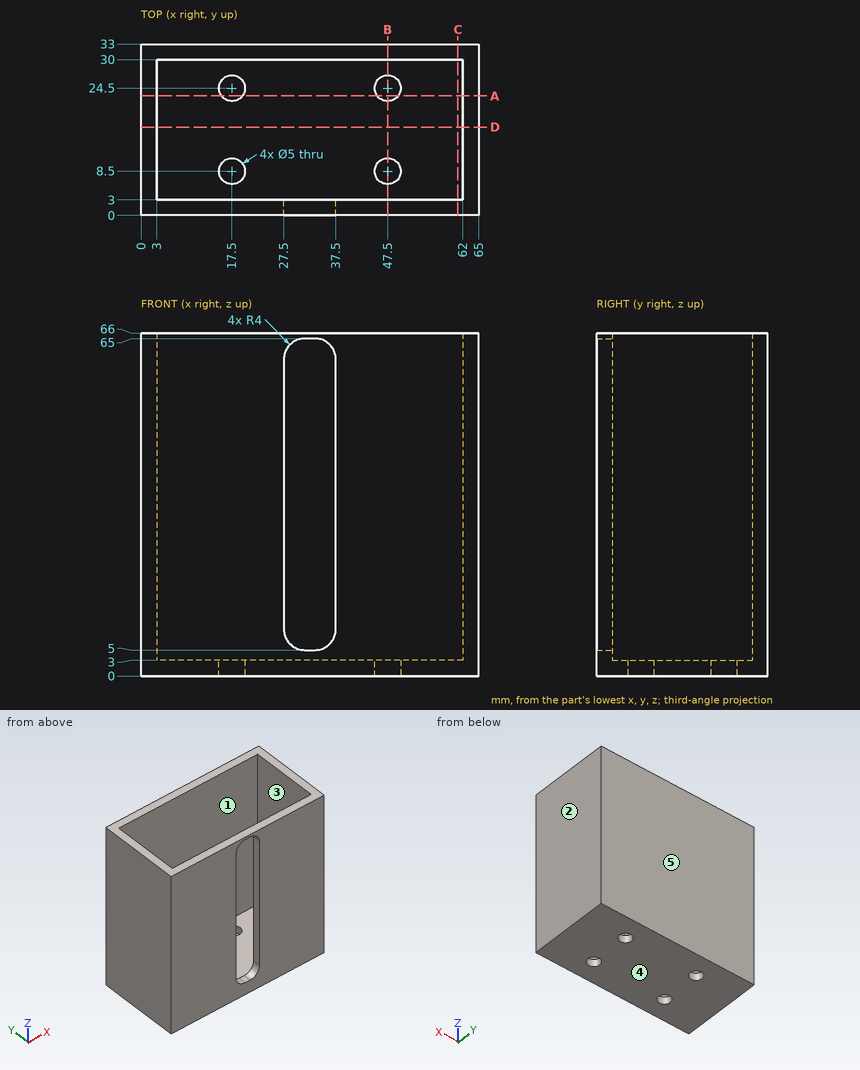
Print and shaded views of the part. All mm, measured from the part's lowest x, y and z. A direction names the side the tool comes from. Round coordinates to 2 decimals unless told otherwise and drop trailing zeros. Write each loop counter-clockwise with the first axis right and the second up, starting at its lowest first coordinate (ties: lowest second). Pieces come first, ordered by that corner, then holes. Notation, with made-up numbers: (83.5, 13) -> (131.5, 13) arc R33 ccw to (131.5, 51) -> close; hole circle Ø7 at (-10.75, 88). An arc over 180 degrees is marked (long way). Return JSON: item names as keys, results as strings. Group by question number.
Q1. Pin check, flat tips, straight feed: pin 1 (8 mm diameter, centred on x = 47.5, y = 24.5, fed in from +Z); pin 2 (4.5 mm diameter, centred on x = 47.5, y = 8.5, fed in from -Z). Stop position of each tip, or through.
Q2. Saw through at D-D on y = 17. Write the cut outline in (x, z).
Q3. Saw through at A-A on y = 23. Write the cut outline in (x, z), plus the area to 3 significant figures.
Q4. Saw through at B-B on x = 47.5. Write the cut outline in (y, z).
Q5. Saw through at C-C on x = 61. Write the cut outline in (y, z).
Q6. Which spindle directions (+Z, -Z, +X, -X, +Y, -Y) get a long thin tool onto all of the face, cutting with end or side? Do the marked faces 1 and 2. Say none if no direction does.
Q7. Mould opens along Y. For the marked faces 3, 4 and 5 say: pulls with the +Y half, pulls with the -Y half, needs draft (parallel to the pull), parting line crosses it, or undercut.
Q8. Probe L1, parallel to Y at x = 17.5, z = 2.1; L2, parallel to X at y = 27.5, z = 37; L3, parallel to Y at x = 47, z = 1. List the from-to ranges inside material, lowest first. Write a range as [from, to].
Answer:
{
 "1": {"pin 1": "z = 3", "pin 2": "through"},
 "2": {"outline": "(0, 0) -> (65, 0) -> (65, 66) -> (62, 66) -> (62, 3) -> (3, 3) -> (3, 66) -> (0, 66) -> close"},
 "3": {"outline": "(0, 0) -> (15.5, 0) -> (15.5, 3) -> (3, 3) -> (3, 66) -> (0, 66) -> close; (19.5, 0) -> (45.5, 0) -> (45.5, 3) -> (19.5, 3) -> close; (49.5, 0) -> (65, 0) -> (65, 66) -> (62, 66) -> (62, 3) -> (49.5, 3) -> close", "area": "549 mm2"},
 "4": {"outline": "(0, 0) -> (6, 0) -> (6, 3) -> (3, 3) -> (3, 66) -> (0, 66) -> close; (11, 0) -> (22, 0) -> (22, 3) -> (11, 3) -> close; (27, 0) -> (33, 0) -> (33, 66) -> (30, 66) -> (30, 3) -> (27, 3) -> close"},
 "5": {"outline": "(0, 0) -> (33, 0) -> (33, 66) -> (30, 66) -> (30, 3) -> (3, 3) -> (3, 66) -> (0, 66) -> close"},
 "6": {"face 1": "+Z", "face 2": "+Z, -Z, +X, +Y, -Y"},
 "7": {"face 3": "undercut", "face 4": "needs draft", "face 5": "pulls with the +Y half"},
 "8": {"L1": "[0, 6], [11, 22], [27, 33]", "L2": "[0, 3], [62, 65]", "L3": "[0, 6.05], [10.95, 22.05], [26.95, 33]"}
}
